```python
from build123d import *

# Parameters (mm, degrees)
CUT_EXTRUDE1_START = 5.5626
CUT_EXTRUDE1_DEPTH = 27.0002
CIRPATTERN1_COUNT  = 14


with BuildPart() as part:
    # Sketch2 → Revolve1 (revolve)
    with BuildSketch(Plane(origin=(0, 0, 0), x_dir=(0, 0, -1), z_dir=(1, 0, 0))):
        with BuildLine():
            Line((-24.6126, 7.9375), (24.6126, 7.9375))
            Line((24.6126, 7.9375), (24.6126, 31.5468))
            Line((24.6126, 31.5468), (23.0251, 31.5468))
            ThreePointArc((23.0251, 31.5468), (21.87887746, 30.758520647), (21.4376, 29.439246357))
            Line((21.4376, 29.439246357), (21.4376, 27.331692713))
            Line((21.4376, 27.331692713), (-5.5626, 27.331692713))
            Line((-5.5626, 27.331692713), (-5.5626, 29.439246357))
            ThreePointArc((-5.5626, 29.439246357), (-6.00387746, 30.758520647), (-7.1501, 31.5468))
            Line((-7.1501, 31.5468), (-8.7376, 31.5468))
            Line((-8.7376, 31.5468), (-8.7376, 19.05))
            Line((-8.7376, 19.05), (-24.6126, 19.05))
            Line((-24.6126, 19.05), (-24.6126, 7.9375))
        make_face()
    revolve(axis=Axis((0, 0, 24.6126), (0, 0, -1)))

    # Sketch3 → Cut-Extrude1 (cut)
    with BuildSketch(Plane.XY.offset(CUT_EXTRUDE1_START)):
        with BuildLine():
            Line((-2.228664044, 24.87377802), (2.228664044, 24.87377802))
            Line((2.228664044, 24.87377802), (3.0607, 27.15977802))
            ThreePointArc((3.0607, 27.15977802), (0, 27.331692713), (-3.0607, 27.15977802))
            Line((-3.0607, 27.15977802), (-2.228664044, 24.87377802))
        make_face()
    cut_extrude1 = extrude(amount=-CUT_EXTRUDE1_DEPTH, mode=Mode.SUBTRACT)

    # CirPattern1: Cut-Extrude1 ×14 about axis
    cirpattern1_axis = Axis((0, 0, 0), (0, 0, 1))
    for i in range(1, CIRPATTERN1_COUNT):
        add(cut_extrude1.rotate(cirpattern1_axis, i * 360 / CIRPATTERN1_COUNT), mode=Mode.SUBTRACT)


solid = part.part
```
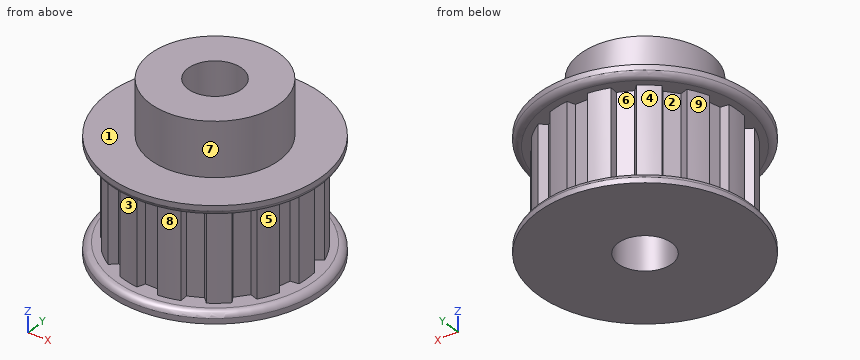
Part model, mm, in its own coordinate system. Face numbers are marked on the shaded views. A direction names the side the tool comes from. Coordinates: 2 decimals unless noted, no trailing zeros. Write each loop counter-clockwise with the first axis right and the second up, starting at its lowest first coordinate (ties: lowest second). Pieces come first, ordered by that corner, then holes.
Item 1: Which spindle directions (+Z, -Z, +X, -X, +Y, -Y) get a long thin tool onto all of the face, cutting with end or side? Do the marked faces 1, 2, 3, 4 and 5. Say none if no direction does.
Item 2: Mould opens along X. For the marked faces 6, 7, 8 and 9 say: released by +X, released by -X, zero draft, split by the parting line, or undercut.
Item 3: Slice it at A-A (y = 0). Write the cut outline in (x, z).
Item 4: Pin check, flat tips, straight feed: pin 1 (5 mm diameter, centred on x = 1, z = -9, fed in from +Y); pin 2 (12 mm diameter, centred on x = 3, z = 9, fed in from -Y); pin 3 (5 mm diameter, centred on y = 16, z = 7, fed in from +X); pin 4 (8 mm diameter, centred on x = -16, z = 17.5, fed in from -Y). Stop position of each tip, or through.
Item 5: Probe line 1 (X direction, y = 0, z = 13); line 2 (Z direction, x = 21, y = 16.5); line 3 (Z direction, x = -25, y = 9). List the from-to ranges inside material, lowest first.
Item 6: Slice it at B-B (x = 0). Write the cut outline in (y, z).
Results found:
1. face 1: +Z
1. face 2: none
1. face 3: -X, -Y
1. face 4: -X, +Y
1. face 5: +X, -Y
2. face 6: undercut
2. face 7: split by the parting line
2. face 8: released by +X
2. face 9: released by -X
3. outline: (-31.55, -24.61) - (-7.94, -24.61) - (-7.94, 24.61) - (-19.05, 24.61) - (-19.05, 8.74) - (-31.55, 8.74) - (-31.55, 7.15) arc R2.19 ccw to (-29.44, 5.56) - (-27.33, 5.56) - (-27.33, -21.44) - (-29.44, -21.44) arc R2.19 ccw to (-31.55, -23.03) - close; (7.94, -24.61) - (31.55, -24.61) - (31.55, -23.03) arc R2.19 ccw to (29.44, -21.44) - (27.33, -21.44) - (27.33, 5.56) - (29.44, 5.56) arc R2.19 ccw to (31.55, 7.15) - (31.55, 8.74) - (19.05, 8.74) - (19.05, 24.61) - (7.94, 24.61) - close
4. pin 1: stops at y = 27.16
4. pin 2: stops at y = -31.55
4. pin 3: stops at x = 28.51
4. pin 4: stops at y = -14.8
5. line 1: x = -19.05 to -7.94, 7.94 to 19.05
5. line 2: z = -24.61 to -21.44, 5.56 to 8.74
5. line 3: z = -24.61 to 8.74
6. outline: (-31.55, -24.61) - (-7.94, -24.61) - (-7.94, 24.61) - (-19.05, 24.61) - (-19.05, 8.74) - (-31.55, 8.74) - (-31.55, 7.15) arc R2.19 ccw to (-29.44, 5.56) - (-24.87, 5.56) - (-24.87, -21.44) - (-29.44, -21.44) arc R2.19 ccw to (-31.55, -23.03) - close; (7.94, -24.61) - (31.55, -24.61) - (31.55, -23.03) arc R2.19 ccw to (29.44, -21.44) - (24.87, -21.44) - (24.87, 5.56) - (29.44, 5.56) arc R2.19 ccw to (31.55, 7.15) - (31.55, 8.74) - (19.05, 8.74) - (19.05, 24.61) - (7.94, 24.61) - close
